Input: part model. Units: mm. Frame: model coordinates. Face numbers are marked on the shaded views. A direction names the side the tool comes from. Round coordinates to 2 decimals unless told otherwise and drop trailing zeros. Loops run counter-clockwise (first coordinate to the right, second up) from the corner with the lowest first, then second, coordinate; pieces in that order, holes last. Notation, with made-up numbers: M 59,34.5 L 116,34.5 A30 cw 116,60.5 Z; hole C 83.25,11.25 d7. An arc over 180 degrees is marked long. Return JSON: item names as keys, results as strings. Group by question number.
1) Contact query for flat-ended pins moving along their axis: P1, Ø3.5, axis at y = 12, z = -7.5, coming from the -X side; P2, Ø3, axis at x = 8, y = 8.5, coming from the -Z side; P3, Ø4, axis at x = -26, z = -6.5, coming from the -Y side; P4, Ø12, axis at x = -26, z = 24, coming from the -Y side. Output: stop coordinate, or through.
2) Section C-C (y = 20.75). Output: boundary loops of the cut face in (x, z), plus the area to 3 significant figures.
3) Section A-A (y = 15). Output: boundary loops of the cut face in (x, z), plus the area to 3 significant figures.
4) Access query for the marked faces 1 and 2. Directions: +Z, -Z, +X, -X, +Y, -Y. A direction counts if a zero-diameter tool reaches every point of the face in a straight line with its end or side. Return the directions, or none.
5) Section B-B (y = 9.5). Count the separate pieces of the cut face and the enclosed holes in it, plus the area to 3 significant figures.
6) Material intervals for line 1 (X direction, y = 5.5, z = 2); line 2 (X direction, y = 17, z = 0); line 3 (X direction, y = 7, z = 0), sorted ascending. Write a range as from..to.
from build123d import *

# Parameters (mm, degrees)
SKETCH_3_W      = 2.4
SKETCH_3_H      = 21.6
SKETCH_4_W      = 1
SKETCH_4_H      = 3
EXTRUDE_1_DEPTH = 16
EXTRUDE_START   = 12
EXTRUDE_2_DEPTH = 12


with BuildPart() as part:
    # 草图3 → 旋转2 (revolve)
    with BuildSketch(Plane.XY, mode=Mode.PRIVATE) as revolve_2_sk:
        with Locations((2.7, 12.8)):
            Rectangle(SKETCH_3_W, SKETCH_3_H)
        Polygon((0, 2), (0, 0), (35, 0), (35, 2), (3.9, 2), (1.5, 2), align=None)
        with BuildLine():
            ThreePointArc((36, 2), (35.5, 2.5), (35, 2))
            Line((35, 2), (36, 2))
        make_face()
        with BuildLine():
            Line((36, 2), (35, 2))
            ThreePointArc((35, 2), (35.5, 1.5), (36, 2))
        make_face()
        with BuildLine():
            ThreePointArc((36, 2), (35.5, 2.5), (35, 2))
            Line((35, 2), (36, 2))
        make_face()
        with BuildLine():
            Line((36, 2), (35, 2))
            ThreePointArc((35, 2), (35.5, 1.5), (36, 2))
        make_face()
        with BuildLine():
            Line((35, 2), (35, 0))
            ThreePointArc((35, 0), (35.5, 0.5), (36, 0))
            Line((36, 0), (36, 2))
            ThreePointArc((36, 2), (35.5, 1.5), (35, 2))
        make_face()
        with BuildLine():
            ThreePointArc((36, 0), (35.5, 0.5), (35, 0))
            Line((35, 0), (36, 0))
        make_face()
        with BuildLine():
            Line((36, 0), (35, 0))
            ThreePointArc((35, 0), (35.5, -0.5), (36, 0))
        make_face()
        with BuildLine():
            ThreePointArc((36, 0), (35.5, 0.5), (35, 0))
            Line((35, 0), (36, 0))
        make_face()
        with BuildLine():
            Line((36, 0), (35, 0))
            ThreePointArc((35, 0), (35.5, -0.5), (36, 0))
        make_face()
    revolve(revolve_2_sk.sketch.rotate(Axis((0, 2, 0), (0, 1, 0)), 90), axis=Axis((0, 2, 0), (0, 1, 0)))

    # 草图4 → 凸台-拉伸1 (add)
    with BuildSketch(Plane(origin=(0, 2, 0), x_dir=(1, 0, 0), z_dir=(0, 1, 0))):
        with Locations((-5.5, 7.25)):
            Rectangle(SKETCH_4_W, SKETCH_4_H)
        Polygon((-6, 4.75), (-5, 4.75), (5, 4.75), (6, 4.75), (6, 5.75), (5, 5.75), (-5, 5.75), (-6, 5.75), align=None)
        with Locations((5.5, 7.25)):
            Rectangle(SKETCH_4_W, SKETCH_4_H)
        Polygon((5, -4.75), (-5, -4.75), (-6, -4.75), (-6, -5.75), (-5, -5.75), (5, -5.75), (6, -5.75), (6, -4.75), align=None)
        with Locations((-5.5, -7.25)):
            Rectangle(SKETCH_4_W, SKETCH_4_H)
        with Locations((5.5, -7.25)):
            Rectangle(SKETCH_4_W, SKETCH_4_H)
    extrude(amount=EXTRUDE_1_DEPTH)

    # 草图6 → 凸台-拉伸2 (add)
    with BuildSketch(Plane(origin=(0, 2, 0), x_dir=(1, 0, 0), z_dir=(0, 1, 0)).offset(EXTRUDE_START)):
        Polygon((-5, -0.5), (-5, 0.5), (-5, 4.75), (-6, 4.75), (-6, -4.75), (-5, -4.75), align=None)
        with BuildLine():
            ThreePointArc((0.5, -3.867815921), (0, -3.9), (-0.5, -3.867815921))
            Line((-0.5, -3.867815921), (-0.5, -4.75))
            Line((-0.5, -4.75), (0.5, -4.75))
            Line((0.5, -4.75), (0.5, -3.867815921))
        make_face()
        with BuildLine():
            Line((-0.5, 4.75), (-0.5, 3.867815921))
            ThreePointArc((-0.5, 3.867815921), (0, 3.9), (0.5, 3.867815921))
            Line((0.5, 3.867815921), (0.5, 4.75))
            Line((0.5, 4.75), (-0.5, 4.75))
        make_face()
        with BuildLine():
            ThreePointArc((-3.867815921, -0.5), (-3.9, 0), (-3.867815921, 0.5))
            Line((-3.867815921, 0.5), (-5, 0.5))
            Line((-5, 0.5), (-5, -0.5))
            Line((-5, -0.5), (-3.867815921, -0.5))
        make_face()
        with BuildLine():
            Line((5, 0.5), (3.867815921, 0.5))
            ThreePointArc((3.867815921, 0.5), (3.891945663, 0.250517372), (3.9, 0))
            ThreePointArc((3.9, 0), (3.891945663, -0.250517372), (3.867815921, -0.5))
            Line((3.867815921, -0.5), (5, -0.5))
            Line((5, -0.5), (5, 0.5))
        make_face()
        Polygon((6, 4.75), (5, 4.75), (5, 0.5), (5, -0.5), (5, -4.75), (6, -4.75), align=None)
    extrude(amount=-EXTRUDE_2_DEPTH)


solid = part.part
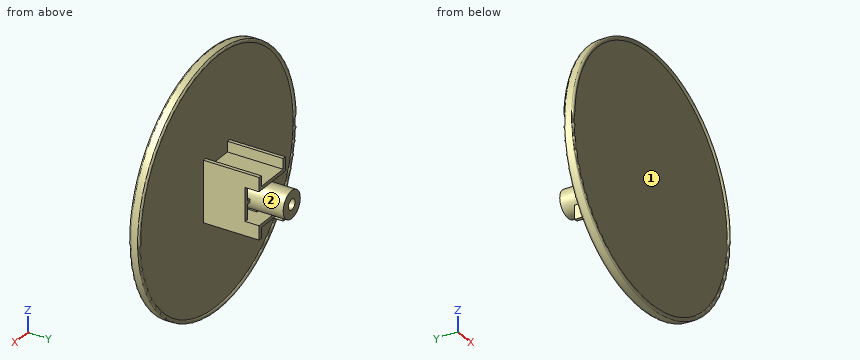
Returned:
{
 "1": {"P1": "stops at x = -6", "P2": "passes through", "P3": "stops at y = 0", "P4": "stops at y = -0.5"},
 "2": {"outline": "C 0,0 d7.8; hole C 0,0 d3", "area": "40.7 mm^2"},
 "3": {"outline": "M -6,-8.75 L -5,-8.75 L -5,-5.75 L 5,-5.75 L 5,-8.75 L 6,-8.75 L 6,-4.75 L -6,-4.75 Z; M -6,4.75 L 6,4.75 L 6,8.75 L 5,8.75 L 5,5.75 L -5,5.75 L -5,8.75 L -6,8.75 Z; C 0,0 d7.8; hole C 0,0 d3", "area": "76.7 mm^2"},
 "4": {"face 1": "-Y", "face 2": "+Y"},
 "5": {"separate pieces": "1", "enclosed holes": "5", "area": "99.7 mm^2"},
 "6": {"line 1": "x = -6..-5, -3.35..3.35, 5..6", "line 2": "x = -3.9..-1.5, 1.5..3.9", "line 3": "x = -6..-1.5, 1.5..6"}
}
